Geometry check sheet. Reference: the model listing, model coordinates, mm. A direction names the side the tool comes from. Coordinates: 2 decimals unless noted, no trailing zeros. Write each loop counter-clockwise with the first axis right and the second up, starting at its lowest first coordinate (ties: lowest second). Pieces come first, ordered by that corner, then holes. Notation, with made-up numbers: M -37,31 L -17,31 A17 ccw -17,50 Z; hole C -31.5,87 d2. An arc over 180 degrees is marked long. Answer as a JSON object with one key per item and string values. Group by question number.
```python
from build123d import *

# Parameters (mm, degrees)
F0_R     = 1.75
F0_R_2   = 8
F1_DEPTH = 6
F3_DEPTH = 3.5


with BuildPart() as f1:
    # F0 (on Top) → F1 (new body)
    with BuildSketch(Plane.XY):
        with BuildLine():
            ThreePointArc((33, 14.4), (31.945584, 16.945584), (29.4, 18))
            Line((29.4, 18), (-29.4, 18))
            ThreePointArc((-29.4, 18), (-31.945584, 16.945584), (-33, 14.4))
            Line((-33, 14.4), (-33, -14.4))
            ThreePointArc((-33, -14.4), (-31.945584, -16.945584), (-29.4, -18))
            Line((-29.4, -18), (29.4, -18))
            ThreePointArc((29.4, -18), (31.945584, -16.945584), (33, -14.4))
            Line((33, -14.4), (33, 14.4))
        make_face()
        with Locations((-26.05, -12.25)):
            Circle(F0_R, mode=Mode.SUBTRACT)
        with Locations((26.05, -12.25)):
            Circle(F0_R, mode=Mode.SUBTRACT)
        with Locations((-13, 0)):
            Circle(F0_R_2, mode=Mode.SUBTRACT)
        with Locations((-26.05, 12.25)):
            Circle(F0_R, mode=Mode.SUBTRACT)
        with Locations((13, 0)):
            Circle(F0_R_2, mode=Mode.SUBTRACT)
        with Locations((26.05, 12.25)):
            Circle(F0_R, mode=Mode.SUBTRACT)
    extrude(amount=F1_DEPTH)

    # F2 (on face) → F3 (cut)
    with BuildSketch(Plane.XY):
        with BuildLine():
            Line((-6, -18), (6, -18))
            Line((6, -18), (6, -5.8))
            ThreePointArc((6, -5.8), (5.648528, -4.951472), (4.8, -4.6))
            Line((4.8, -4.6), (-4.8, -4.6))
            ThreePointArc((-4.8, -4.6), (-5.648528, -4.951472), (-6, -5.8))
            Line((-6, -5.8), (-6, -18))
        make_face()
        with BuildLine():
            ThreePointArc((4.8, 4.6), (5.648528, 4.951472), (6, 5.8))
            Line((6, 5.8), (6, 18))
            Line((6, 18), (-6, 18))
            Line((-6, 18), (-6, 5.8))
            ThreePointArc((-6, 5.8), (-5.648528, 4.951472), (-4.8, 4.6))
            Line((-4.8, 4.6), (4.8, 4.6))
        make_face()
    extrude(amount=F3_DEPTH, mode=Mode.SUBTRACT)


solid = f1.part
```
1) Section check C-C (y = 0). Record the cut outline in (x, z), then the cut area to 3 significant figures.
2) Material ranges on probe 1 along Y at (x, z) = (-26.05, 2.5); probe 2 along X at (y, z) = (-5.5, 3.95); probe 3 along X at (y, z) = (1.5, 5.6), recorded low to high. Write a range as [from, to].
3) Draft check along X on faces 4 (the flat face through (0, 0, 0)), 5 (the cylindrical face through (31.97, 16.92, 2.96)), 6 (the flat face through (6, 12, 2)), 7 (the flat face through (-33, 0, 3)). Enter one of: +X half, -X half, draft (parallel to the pull), parting line (faces both ways), or undercut.
4) Set-up check for faces 1 (the flat face through (0, -11, 3.5)), 2 (the cylindrical face through (5.639, 4.942, 1.726)), 3 (the flat face through (0, -18, 4)): record each of +Z, -Z, +X, -X, +Y, -Y from which the full face is reachable in a straight line by a thin tool's end or side.
5) Go/stop test with flat-tipped pins: pin 1 Ø8 at (x, y) = (14, 2.5) entering from +Z; pin 2 Ø6 at (x, y) = (-2.5, -13.5) entering from -Z; pin 3 Ø1 at (x, z) = (1.5, 1.5) entering from -Y. Record where each tip stops, or that it passes through.
6) Section check A-A (x = -26.05). Record the cut outline in (y, z).
7) Section check D-D (x = -13). Record the cut outline in (y, z), then the cut area to 3 significant figures.
8) Section check B-B (z = 0.95). Record the cut outline in (x, y), then the cut area to 3 significant figures.
Entries:
{
 "1": {"outline": "M -33,0 L -21,0 L -21,6 L -33,6 Z; M -5,0 L 5,0 L 5,6 L -5,6 Z; M 21,0 L 33,0 L 33,6 L 21,6 Z", "area": "204 mm^2"},
 "2": {"probe 1": "[-18, -14], [-10.5, 10.5], [14, 18]", "probe 2": "[-33, -18.81], [-7.19, 7.19], [18.81, 33]", "probe 3": "[-33, -20.86], [-5.14, 5.14], [20.86, 33]"},
 "3": {"face 4": "draft", "face 5": "+X half", "face 6": "undercut", "face 7": "-X half"},
 "4": {"face 1": "-Z, -Y", "face 2": "-Z, +Y", "face 3": "+Z, -Z, +X, -X, -Y"},
 "5": {"pin 1": "through", "pin 2": "z = 3.5", "pin 3": "y = -4.6"},
 "6": {"outline": "M -18,0 L -14,0 L -14,6 L -18,6 Z; M -10.5,0 L 10.5,0 L 10.5,6 L -10.5,6 Z; M 14,0 L 18,0 L 18,6 L 14,6 Z"},
 "7": {"outline": "M -18,0 L -8,0 L -8,6 L -18,6 Z; M 8,0 L 18,0 L 18,6 L 8,6 Z", "area": "120 mm^2"},
 "8": {"outline": "M -33,-14.4 A3.6 ccw -29.4,-18 L -6,-18 L -6,-5.8 A1.2 cw -4.8,-4.6 L 4.8,-4.6 A1.2 cw 6,-5.8 L 6,-18 L 29.4,-18 A3.6 ccw 33,-14.4 L 33,14.4 A3.6 ccw 29.4,18 L 6,18 L 6,5.8 A1.2 cw 4.8,4.6 L -4.8,4.6 A1.2 cw -6,5.8 L -6,18 L -29.4,18 A3.6 ccw -33,14.4 Z; hole C -26.05,-12.25 d3.5; hole C -26.05,12.25 d3.5; hole C -13,0 d16; hole C 13,0 d16; hole C 26.05,-12.25 d3.5; hole C 26.05,12.25 d3.5", "area": "1,600 mm^2"}
}
